```python
from build123d import *

# Parameters (mm, degrees)
SKETCH1_R           = 6
BOSS_EXTRUDE1_DEPTH = 10
BOSS_EXTRUDE2_START = 8
SKETCH3_R           = 6
BOSS_EXTRUDE2_DEPTH = 8


with BuildPart() as part:
    # Sketch1 → Boss-Extrude1 (new body)
    with BuildSketch(Plane.XY):
        with BuildLine():
            Line((-35, 13), (35, 13))
            ThreePointArc((35, 13), (48, 0), (35, -13))
            Line((35, -13), (-35, -13))
            ThreePointArc((-35, -13), (-48, 0), (-35, 13))
        make_face()
        with Locations((-35, 0)):
            Circle(SKETCH1_R, mode=Mode.SUBTRACT)
        with Locations((35, 0)):
            Circle(SKETCH1_R, mode=Mode.SUBTRACT)
    extrude(amount=BOSS_EXTRUDE1_DEPTH)

    # Sketch3 → Boss-Extrude2 (add)
    with BuildSketch(Plane(origin=(0, 0, 0), x_dir=(0, 0, -1), z_dir=(1, 0, 0)).offset(BOSS_EXTRUDE2_START)):
        with BuildLine():
            Line((-10, -13), (-29, -13))
            ThreePointArc((-29, -13), (-42, 0), (-29, 13))
            Line((-29, 13), (-10, 13))
            Line((-10, 13), (-10, -13))
        make_face()
        with Locations((-29, 0)):
            Circle(SKETCH3_R, mode=Mode.SUBTRACT)
    boss_extrude2 = extrude(amount=BOSS_EXTRUDE2_DEPTH)

    # Mirror1: Boss-Extrude2 across plane
    add(boss_extrude2.mirror(Plane(origin=(0, 0, 0), x_dir=(0, 0, 1), z_dir=(1, 0, 0))))


solid = part.part
```
Work out the finished part from the listing and answer in its coordinate system (mm). A direction names the side the tool comes from. Round coordinates to 2 decimals unless told otherwise and drop trailing zeros. Loops run counter-clockwise (first coordinate to the right, second up) from the corner with the lowest first, then second, coordinate; pieces in that order, holes last. Notation, with made-up numbers: M 34.25,67 L 45.25,67 A32 cw 45.25,101 Z; hole C 69.5,76 d2. An arc over 180 degrees is marked long. One line per question, with ' | ' between items.
Q1. Find section C-C, the plane x = -36. Give the vertices of the cut face in (y, z).
Conclusion:
outline: M -12.96,0 L -5.92,0 L -5.92,10 L -12.96,10 Z; M 5.92,0 L 12.96,0 L 12.96,10 L 5.92,10 Z
Q2. Find section A-A, the plane y = 0. Give the vertices of the cut face in (x, z).
Conclusion:
outline: M -48,0 L -41,0 L -41,10 L -48,10 Z; M -29,0 L 29,0 L 29,10 L 16,10 L 16,23 L 8,23 L 8,10 L -8,10 L -8,23 L -16,23 L -16,10 L -29,10 Z; M -16,35 L -8,35 L -8,42 L -16,42 Z; M 8,35 L 16,35 L 16,42 L 8,42 Z; M 41,0 L 48,0 L 48,10 L 41,10 Z
Q3. Each of these flat-tipped pins is pushed along its axis until it touches: pin 1 Ø11 at (x, y) = (35, 0) entering from -Z; pin 2 Ø15.5 at (x, y) = (-35, 0) entering from +Z; pin 3 Ø1.5 at (y, z) = (-10, 8) entering from +X; pin 4 Ø6 at (y, z) = (4.5, 26.5) entering from -X. Where does it stop, or does it pass through?
Conclusion:
pin 1: passes through | pin 2: stops at z = 10 | pin 3: stops at x = 44.13 | pin 4: stops at x = -16
Q4. Consider line 1 along X through (y, z) = (4, 19); line 2 along Y through (x, z) = (-10, 29); line 3 along Z through (x, y) = (0, 4). Determine where each line is inside the solid, lowest interval first. Write a range as from..to.
Conclusion:
line 1: x = -16..-8, 8..16 | line 2: y = -13..-6, 6..13 | line 3: z = 0..10
Q5. The mould has two halves that part along Y. Classify faces 5 (the cylindrical face through (30.24, -3.65, 4.93)), 6 (the cylindrical face through (-12, 0, 42)), 7 (the flat face through (1, 0, 0)): +Y half, -Y half, draft (parallel to the pull), parting line (faces both ways), or undercut.
Conclusion:
face 5: undercut | face 6: parting line | face 7: draft
Q6. Find section D-D, the plane x = 11. Give the vertices of the cut face in (y, z), then the cut area to 3 significant figures.
Conclusion:
outline: M -13,0 L 13,0 L 13,29 A13 ccw -13,29 Z; hole C 0,29 d12 | area: 906 mm2
Q7. Find section B-B, the plane z = 17. Give the vertices of the cut face in (x, y).
Conclusion:
outline: M -16,-13 L -8,-13 L -8,13 L -16,13 Z; M 8,-13 L 16,-13 L 16,13 L 8,13 Z
Q8. A tool of negligible diameter and unlimited length cuts with its end or side. For faces 1 (the flat face through (-16, 0, 22)), 2 (the flat face through (0, 0, 10)), 3 (the flat face through (28.7, 0.2, 10)), 4 (the cylindrical face through (-41, 0, 5)), from which of +Z, -Z, +X, -X, +Y, -Y can it reach the whole face along a straight path? Write none if from no direction.
Conclusion:
face 1: +Z, -X, +Y, -Y | face 2: +Z, +Y, -Y | face 3: +Z, +X, +Y, -Y | face 4: +Z, -Z
